Geometry: see drawing. Coordinates: mm, zero at the bounding-box minimum. Coordinates: 2 decimals unless noted, no trailing zeros. Loops run counter-clockwise (first coordinate to the right, second up) from the corner with the lowest first, then second, coordinate; pieces in that order, holes last. Notation, with made-up numbers: (-33.75, 22.25) -> (-21.75, 22.25) arc R14 ccw to (-21.75, 46.25) -> close; hole circle Ø5 at (43.25, 13.5). An arc over 180 degrees is marked (long way). One line per item, written item: value. Start each with the question number.
Item 1: Ray query, probe 1 along Y at (x, z) = (0.4, 22); probe 2 along Z at (x, y) = (1.05, 23.75) (1 decimal); probe 3 along Y at (x, z) = (1.75, 19.75). Return the intervals inside material, ascending. Write a range as from..to.
Item 2: Section query C-C on y = 18.25. Return loops of the section in (x, z).
Item 3: Section query B-B on z = 7.25. Return loops of the section in (x, y).
Item 4: Section query A-A on x = 0.35. Return loops of the section in (y, z), then the cut area to 3 significant figures.
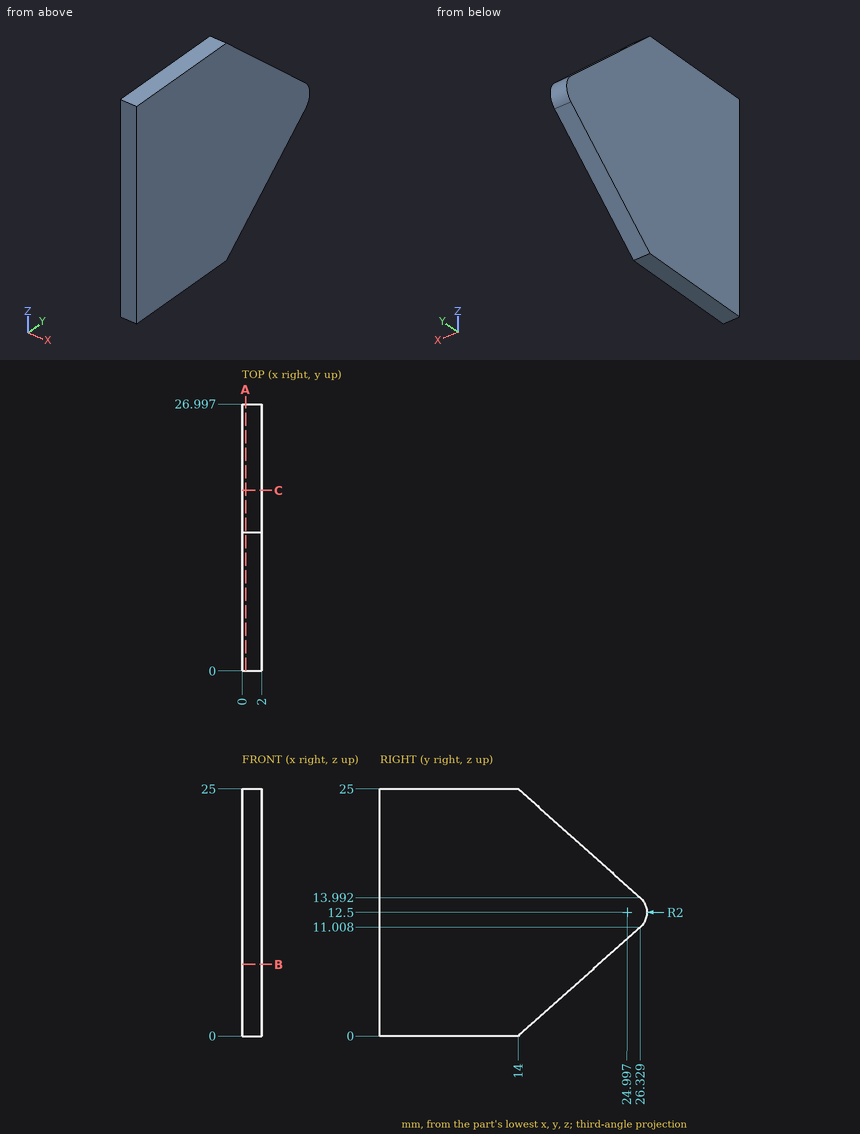
Reply:
1. probe 1: y = 0..17.36
1. probe 2: z = 8.7..16.3
1. probe 3: y = 0..19.88
2. outline: (0, 3.79) -> (2, 3.79) -> (2, 21.21) -> (0, 21.21) -> close
3. outline: (0, 0) -> (2, 0) -> (2, 22.12) -> (0, 22.12) -> close
4. outline: (0, 0) -> (14, 0) -> (26.33, 11.01) arc R2 ccw to (26.33, 13.99) -> (14, 25) -> (0, 25) -> close
4. area: 524 mm²
